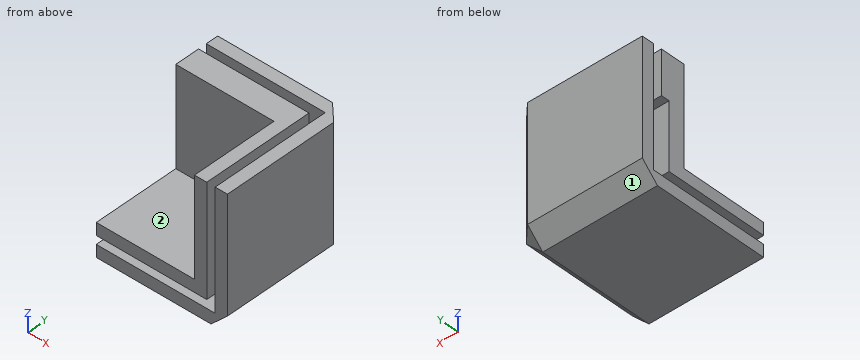
from build123d import *

# Parameters (mm, degrees)
SKETCH4_W               = 50.8
SKETCH4_H               = 50.8
BOSS_EXTRUDE4_DEPTH     = 50.8
SKETCH5_W               = 38.0238
SKETCH5_H               = 38.0238
CUT_EXTRUDE1_DEPTH      = 38.0238
CUT_EXTRUDE2_DEPTH      = 31.6738
CUT_EXTRUDE3_DEPTH      = 88.988181024
CUT_EXTRUDE3_DEPTH_BACK = 31.6738
CUT_EXTRUDE4_DEPTH      = 31.6738
CHAMFER1_SIZE           = 6.35
SKETCH9_W               = 38.0238
SKETCH9_H               = 4.7625
BOSS_EXTRUDE5_DEPTH     = 38.0238
SKETCH10_W              = 25.781
SKETCH10_H              = 3.2258
CUT_EXTRUDE5_DEPTH      = 31.6738


with BuildPart() as part:
    # Sketch4 → Boss-Extrude4 (new body)
    with BuildSketch(Plane(origin=(0, 0, 0), x_dir=(1, 0, 0), z_dir=(0, 1, 0))):
        with Locations((25.4, 25.4)):
            Rectangle(SKETCH4_W, SKETCH4_H)
    extrude(amount=BOSS_EXTRUDE4_DEPTH)

    # Sketch5 → Cut-Extrude1 (cut)
    with BuildSketch(Plane.XZ):
        with Locations((19.0119, -19.0119)):
            Rectangle(SKETCH5_W, SKETCH5_H)
    extrude(amount=-CUT_EXTRUDE1_DEPTH, mode=Mode.SUBTRACT)

    # Sketch6 → Cut-Extrude2 (cut)
    with BuildSketch(Plane.ZY):
        Polygon((-46.0375, 0), (-42.7863, 0), (-42.7863, 42.7863), (0, 42.7863), (0, 46.0375), (-46.0375, 46.0375), align=None)
    extrude(amount=-CUT_EXTRUDE2_DEPTH, mode=Mode.SUBTRACT)

    # Sketch7 → Cut-Extrude3 (cut, two sides: drawn at the far end of the back side and taken through both)
    with BuildSketch(Plane.XY.offset(-CUT_EXTRUDE3_DEPTH_BACK)):
        Polygon((46.0375, 46.0375), (31.6738, 46.0375), (31.6738, 42.7863), (42.7863, 42.7863), (42.7863, 0), (46.0375, 0), align=None)
    extrude(amount=CUT_EXTRUDE3_DEPTH + CUT_EXTRUDE3_DEPTH_BACK, mode=Mode.SUBTRACT)

    # Sketch8 → Cut-Extrude4 (cut)
    with BuildSketch(Plane.XZ):
        Polygon((31.6738, -46.0375), (46.0375, -46.0375), (46.0375, -31.6738), (42.7863, -31.6738), (42.7863, -42.7863), (31.6738, -42.7863), align=None)
    extrude(amount=-CUT_EXTRUDE4_DEPTH, mode=Mode.SUBTRACT)

    # Chamfer1
    chamfer1_edges = [part.edges().sort_by_distance(p)[0] for p in [
        (50.8, 50.8, -25.4),
        (25.4, 50.8, -50.8),
        (50.8, 25.4, -50.8),
    ]]
    chamfer(chamfer1_edges, length=CHAMFER1_SIZE)

    # Sketch9 → Boss-Extrude5 (add)
    with BuildSketch(Plane.ZY.offset(-38.0238)):
        with Locations((-19.0119, 35.64255)):
            Rectangle(SKETCH9_W, SKETCH9_H)
    extrude(amount=BOSS_EXTRUDE5_DEPTH)

    # Sketch10 → Cut-Extrude5 (cut)
    with BuildSketch(Plane.ZY):
        with Locations((-29.8958, 41.1734)):
            Rectangle(SKETCH10_W, SKETCH10_H)
    extrude(amount=-CUT_EXTRUDE5_DEPTH, mode=Mode.SUBTRACT)


solid = part.part
Geometry: final body of the model. Coordinates: model frame, mm. Face numbers are marked on the shaded views. A direction names the side the tool comes from. Round coordinates to 2 decimals unless told otherwise and drop trailing zeros. Order: outer loops, then holes, each group sorted by start corner. A loop starts at its lowest first (then second) coordinate and runs counter-clockwise, first axis right, second up. Notation, with made-up numbers: (19, 7.5) - (68, 7.5) arc R27 ccw to (68, 45.5) - close; hole circle Ø2 at (75.5, -1.5). An arc over 180 degrees is marked (long way). Write each question's results on one line, items separated by ' | '.
Item 1: Reachability of the marked faces 1 and 2 from +Z, -Z, +X, -X, +Y, -Y: full face, straight path, thin tool, end or side. Return the list, or none.
Completed:
face 1: -Z, +X, -X, +Y | face 2: +Z, -X, -Y
Item 2: Section B-B, the plane x = 8. Return the cut outline in (y, z).
Completed:
outline: (0, -50.8) - (44.45, -50.8) - (50.8, -44.45) - (50.8, 0) - (46.04, 0) - (46.04, -46.04) - (0, -46.04) - close; (0, -42.79) - (39.56, -42.79) - (39.56, -17.01) - (42.79, -17.01) - (42.79, 0) - (33.26, 0) - (33.26, -38.02) - (0, -38.02) - close
Item 3: Section A-A, the plane z = -6.5. Return the cut outline in (x, y).
Completed:
outline: (0, 33.26) - (38.02, 33.26) - (38.02, 0) - (42.79, 0) - (42.79, 42.79) - (0, 42.79) - close; (0, 46.04) - (46.04, 46.04) - (46.04, 0) - (50.8, 0) - (50.8, 44.45) - (44.45, 50.8) - (0, 50.8) - close
Item 4: Material intervals for line 1 along Y through (x, z) = (12, -6); line 2 along Y through (x, z) = (27, -28); line 3 along Z through (x, y) = (11, 38), sorted ascending. Write a range as [from, to].
Completed:
line 1: [33.26, 42.79], [46.04, 50.8] | line 2: [33.26, 39.56], [46.04, 50.8] | line 3: [-50.8, -46.04], [-42.79, 0]
Item 5: First-contact query: pin 1 Ø10 at (x, y) = (25.5, 23.5) entering from +Z; pin 2 Ø3 at (y, z) = (29, -13.5) entering from -X; pin 3 Ø19 at (x, z) = (17, -19) entering from -Y. Flat tips, straight axial feed; report the tip coordinate or a pass-through.
Completed:
pin 1: z = -38.02 | pin 2: x = 38.02 | pin 3: y = 33.26
Item 6: Section D-D, the plane z = -19. Return the cut outline in (x, y), and give its area (3 significant figures).
Completed:
outline: (0, 33.26) - (38.02, 33.26) - (38.02, 0) - (42.79, 0) - (42.79, 42.79) - (31.67, 42.79) - (31.67, 39.56) - (0, 39.56) - close; (0, 46.04) - (46.04, 46.04) - (46.04, 0) - (50.8, 0) - (50.8, 44.45) - (44.45, 50.8) - (0, 50.8) - close | area: 905 mm^2
Item 7: Section C-C, the plane y = 24. Return the cut outline in (x, z), and give its area (3 significant figures).
Completed:
outline: (0, -50.8) - (44.45, -50.8) - (50.8, -44.45) - (50.8, 0) - (46.04, 0) - (46.04, -46.04) - (0, -46.04) - close; (0, -42.79) - (42.79, -42.79) - (42.79, 0) - (38.02, 0) - (38.02, -38.02) - (0, -38.02) - close | area: 826 mm^2
